Drawing for the job (mm, zero at the part's lowest x, y, z). A direction names the side the tool comes from. Coordinates: 2 decimals unless noted, no trailing zeros. Write each loop counter-clockwise with the first axis right and the second up, starting at its lowest first coordinate (ties: lowest second). Pieces come first, ordered by that corner, then holes. Notation, with made-up numbers: M 52,48 L 79,48 A17 ccw 79,76 Z; hole C 10.5,28.25 d2. An arc over 180 degrees is marked long. Use a Markdown table: item, result. Add a question column.
Q1. Slice it at D-D on z = 2.5. Write the cut outline in (x, y), then the cut area to 3 significant figures.
Q2. Tool access for the marked faces 1, 2 and 3: list every direction of +Z, -Z, +X, -X, +Y, -Y with a clear straight run to the whole face (end or side of a thin tool).
Q3. Pin check, flat tips, straight feed: pin 1 Ø1.5 at (x, y) = (10.5, 3) entering from -Z; pin 2 Ø1.8 at (x, z) = (13, 2) entering from +Y; pin 3 Ø3 at (y, z) = (6, 1) entering from -X; pin 4 Ø1.5 at (y, z) = (4.5, 2) entering from +X. Stop position of each tip, or through.
Q4. Mould opens along Z. For the marked faces 4, 5 and 6 say: released by +Z, released by -Z, zero draft, split by the parting line, or undercut.
Q5. Slice it at C-C on z = 0.75. Write the cut outline in (x, y).
Q6. Slice it at B-B on x = 18.5. Write the cut outline in (y, z), then the cut area to 3 significant figures.
Q7. Wall check: L1, parallel to X at y = 7.25, z = 2.25; L2, parallel to X at y = 2.75, z = 4.5; L3, parallel to Z at x = 1.5, y = 7.5. Give the ranges that are in metal, low to high. Write a range as from..to.
Q8. Slice it at A-A on y = 2. Write the cut outline in (x, z).
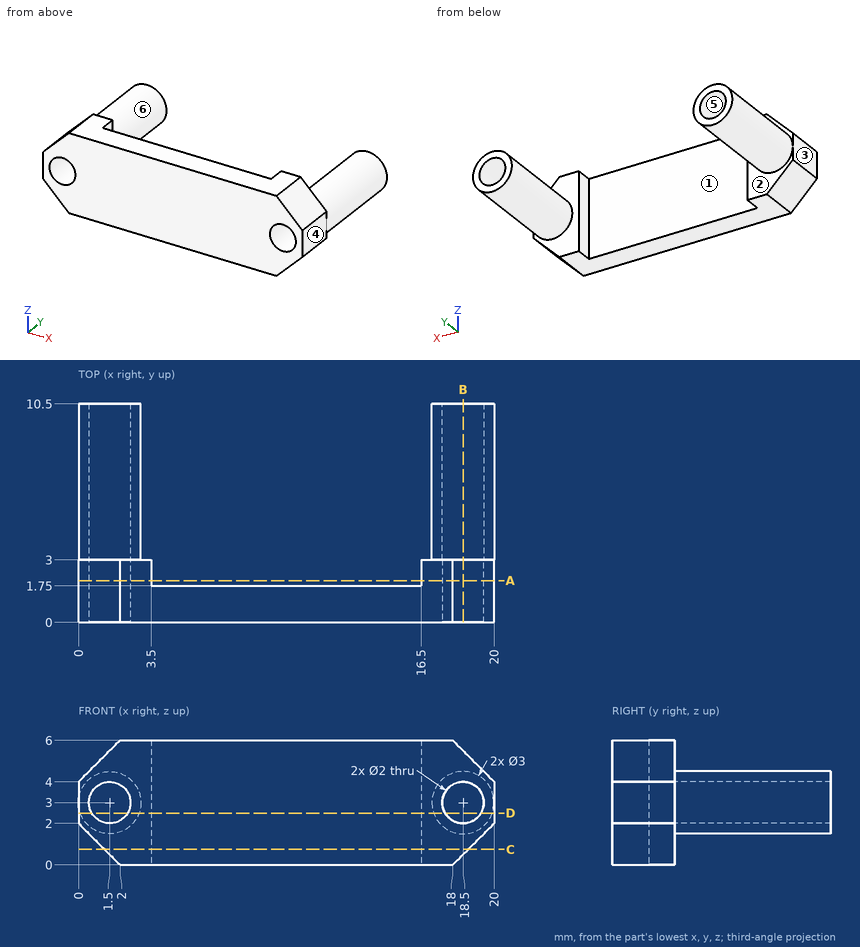
Recorded:
| question | item | result |
|---|---|---|
| 1 | outline | M 0,0 L 0.63,0 L 0.63,10.5 L 0.09,10.5 L 0.09,3 L 0,3 Z; M 2.37,0 L 17.63,0 L 17.63,10.5 L 17.09,10.5 L 17.09,3 L 16.5,3 L 16.5,1.75 L 3.5,1.75 L 3.5,3 L 2.91,3 L 2.91,10.5 L 2.37,10.5 Z; M 19.37,0 L 20,0 L 20,3 L 19.91,3 L 19.91,10.5 L 19.37,10.5 Z |
| 1 | area | 49.8 mm² |
| 2 | face 1 | +Z, -Z, +Y |
| 2 | face 2 | +Y |
| 2 | face 3 | +Z, -Z, -X, +Y, -Y |
| 3 | pin 1 | through |
| 3 | pin 2 | y = 1.75 |
| 3 | pin 3 | x = 0.09 |
| 3 | pin 4 | x = 19.98 |
| 4 | face 4 | zero draft |
| 4 | face 5 | undercut |
| 4 | face 6 | split by the parting line |
| 5 | outline | M 1.25,0 L 18.75,0 L 18.75,3 L 16.5,3 L 16.5,1.75 L 3.5,1.75 L 3.5,3 L 1.25,3 Z |
| 6 | outline | M 0,0.5 L 3,0.5 L 3,1.5 L 10.5,1.5 L 10.5,2 L 0,2 Z; M 0,4 L 10.5,4 L 10.5,4.5 L 3,4.5 L 3,5.5 L 0,5.5 Z |
| 6 | area | 16.5 mm² |
| 7 | L1 | 0.2..0.84, 2.16..2.8, 17.2..17.84, 19.16..19.8 |
| 7 | L2 | 0.5..3.5, 16.5..19.5 |
| 7 | L3 | 1.5..2, 4..4.5 |
| 8 | outline | M 0,2 L 2,0 L 3.5,0 L 3.5,6 L 2,6 L 0,4 Z; M 16.5,0 L 18,0 L 20,2 L 20,4 L 18,6 L 16.5,6 Z; hole C 1.5,3 d2; hole C 18.5,3 d2 |
